Can you work these out from the model? Positions are in its coordinate system, mm. A direction names the side the tool comes from. Round coordinates to 2 decimals unless told otherwise and drop trailing zeros. Loops run counter-clockwise (first coordinate to the right, second up) from the corner with the lowest first, then second, coordinate; pieces in that order, holes last.
(1) I want a section at B-B on y = 3.5. Write out the boundary of the cut face in (x, z).
(2) I want a section at C-C on x = 48.5. Write out the boundary of the cut face in (y, z), plus the area to 3 significant figures.
(3) Will these pins go through, and if not, where does the flat tip stop? pin 1 Ø4 at (x, z) = (6.5, 6) entering from -Y; pin 2 Ø3 at (x, z) = (16, 2.5) entering from +Y; pin 3 Ø1.5 at (y, z) = (15.5, 3) entering from +X; pin 4 Ø12 at (x, y) = (18.5, 8.5) entering from -Z.
(4) I want a section at D-D on x = 25. Write out the boundary of the cut face in (y, z).
(5) Which directions (+Z, -Z, +X, -X, +Y, -Y) give clear straight access to the entire face, cutting with the end or side of a thin tool? Please do faces 1 (the face through (27, 0, 6)), 2 (the face through (7, 5, 3)), 3 (the face through (49, 5, 3)).
(6) I want a section at A-A on z = 6. Write out the boundary of the cut face in (x, y), plus the area to 3 significant figures.
(7) Thinking about a two-plate mould opening in Z: for faces 4 (the face through (54.1, 2.54, 11.14)), 5 (the face through (54.1, 2.54, 0.86)), 6 (the face through (55, 2, 6)), 7 (the face through (5.749, 2.465, 3.615)), which applies, released by +Z, released by -Z, zero draft, split by the parting line, or undercut?
(8) If I drill on line 1 along X through (y, z) = (3.9, 6); line 2 along Y through (x, z) = (27.5, 9.75); line 3 along Z through (x, y) = (48.5, 1.3), over which ranges is the centre line in solid material (lowest first)?
from build123d import *

# Parameters (mm, degrees)
BOSS_EXTRUDE3_DEPTH = 12
SKETCH7_R           = 5.987031074
CUT_EXTRUDE1_DEPTH  = 12
SKETCH9_R           = 2.5
CUT_EXTRUDE2_DEPTH  = 5
FILLET2_R           = 3


with BuildPart() as part:
    # Sketch5 → Boss-Extrude3 (new body)
    with BuildSketch(Plane.XY):
        with BuildLine():
            Line((0, 0), (55, 0))
            Line((55, 0), (55, 5))
            Line((55, 5), (42, 5))
            Line((42, 5), (40, 15))
            ThreePointArc((40, 15), (27.5, 27.5), (15, 15))
            Line((15, 15), (13, 5))
            Line((13, 5), (0, 5))
            Line((0, 5), (0, 0))
        make_face()
    extrude(amount=BOSS_EXTRUDE3_DEPTH)

    # Sketch7 → Cut-Extrude1 (cut)
    with BuildSketch(Plane(origin=(0, 0, 0), x_dir=(-1, 0, 0), z_dir=(0, 0, -1))):
        with Locations((-27.5, 15)):
            Circle(SKETCH7_R)
    extrude(amount=-CUT_EXTRUDE1_DEPTH, mode=Mode.SUBTRACT)

    # Sketch9 → Cut-Extrude2 (cut)
    with BuildSketch(Plane(origin=(0, 0, 0), x_dir=(1, 0, 0), z_dir=(0, 1, 0))):
        with Locations(Location((6.5, -6, 0), (0, 0, 90))):
            Circle(SKETCH9_R)
        with Locations(Location((48.5, -6, 0), (0, 0, 90))):
            Circle(SKETCH9_R)
    extrude(amount=CUT_EXTRUDE2_DEPTH, mode=Mode.SUBTRACT)

    # Fillet2
    fillet2_edges = [part.edges().sort_by_distance(p)[0] for p in [
        (0, 2.5, 0),
        (0, 2.5, 12),
        (55, 2.5, 12),
        (55, 2.5, 0),
    ]]
    fillet(fillet2_edges, radius=FILLET2_R)


solid = part.part
Filled sheet:
1. outline: (0, 3) arc R3 ccw to (3, 0) - (52, 0) arc R3 ccw to (55, 3) - (55, 9) arc R3 ccw to (52, 12) - (3, 12) arc R3 ccw to (0, 9) - close; hole circle Ø5 at (6.5, 6); hole circle Ø5 at (48.5, 6)
2. outline: (0, 0) - (5, 0) - (5, 3.5) - (0, 3.5) - close; (0, 8.5) - (5, 8.5) - (5, 12) - (0, 12) - close
2. area: 35.0 mm2
3. pin 1: passes through
3. pin 2: stops at y = 22.5
3. pin 3: stops at x = 40.05
3. pin 4: stops at z = 0
4. outline: (0, 0) - (9.56, 0) - (9.56, 12) - (0, 12) - close; (20.44, 0) - (27.25, 0) - (27.25, 12) - (20.44, 12) - close
5. face 1: +Z, -Z, +X, -X, -Y
5. face 2: +Z, -Z, -X, +Y
5. face 3: +Z, -Z, +X, +Y
6. outline: (0, 0) - (4, 0) - (4, 5) - (0, 5) - close; (9, 0) - (46, 0) - (46, 5) - (42, 5) - (40, 15) arc R12.5 ccw to (15, 15) - (13, 5) - (9, 5) - close; (51, 0) - (55, 0) - (55, 5) - (51, 5) - close; hole circle Ø11.97 at (27.5, 15)
6. area: 628 mm2
7. face 4: released by +Z
7. face 5: released by -Z
7. face 6: zero draft
7. face 7: undercut
8. line 1: x = 0 to 4, 9 to 46, 51 to 55
8. line 2: y = 0 to 9.01, 20.99 to 27.5
8. line 3: z = 0 to 3.5, 8.5 to 12
